Geometry check sheet. Reference: the model listing, model coordinates, mm. Face numbers are marked on the shaded views. Round coordinates to 2 decimals unless told otherwise and drop trailing zeros. Order: outer loops, then holes, each group sorted by start corner. A loop starts at its lowest first (then second) coordinate and runs counter-clockwise, first axis right, second up.
(1) Sectioned sample at C-C (z = 8). Record the boundary of the cut face in (x, y), plus the area to 3 significant figures.
(2) Sectioned sample at D-D (y = -1.95). Record the boundary of the cut face in (x, z).
(3) Material ranges on line 1 along Y through (x, z) = (8, 5.5); line 2 along X through (y, z) = (-0.45, -12); line 3 along X through (y, z) = (-0.2, 14.5), recorded low to high.
(4) Sectioned sample at A-A (y = 0). Record the boundary of the cut face in (x, z), plus the area to 3 significant figures.
(5) Sectioned sample at B-B (x = 0). Record the boundary of the cut face in (y, z).
(6) Release check for a two-part mould opening along X. For the marked faces 1 and 2 record: +X half, -X half, draft (parallel to the pull), parting line (faces both ways), or undercut.
(7) Go/stop test with flat-tipped pins: pin 1 (1 mm diameter, centred on y = 1.5, z = -7, fed in from -X); pin 2 (1.5 mm diameter, centred on x = 9.5, z = 12, fed in from -Y). Record where each tip stops, or that it passes through.
from build123d import *

# Parameters (mm, degrees)
SKETCH1_R                       = 3
BOSS_EXTRUDE1_DEPTH             = 17.5
M3_CLEARANCE_HOLE_D             = 3.2
BOSS_EXTRUDE2_REACH             = 19.5
SKETCH2_R                       = 3
BOSS_EXTRUDE2_DIRECTION_2_REACH = 19.5
M3_CLEARANCE_HOLE2_D            = 3.2


with BuildPart() as part:
    # Sketch1 → Boss-Extrude1 (new body, symmetric)
    with BuildSketch(Plane.XY):
        Circle(SKETCH1_R)
    extrude(amount=BOSS_EXTRUDE1_DEPTH, both=True)

    # M3 Clearance Hole (through all)
    with Locations(Plane.XY.offset(17.5)):
        with Locations((0, 0)):
            Hole(M3_CLEARANCE_HOLE_D / 2)

    # Boss-Extrude2: up to this face of the body (flat: up to its plane)
    boss_extrude2_end = Plane(part.part.faces().sort_by_distance((-2.915147186, 0, 17.5))[0])
    # Sketch2 → Boss-Extrude2 (add, up to the picked face)
    with BuildSketch(Plane.XY, mode=Mode.PRIVATE) as boss_extrude2_sk1:
        with Locations((8, 0)):
            Circle(SKETCH2_R)
    boss_extrude2_tool1 = split(extrude(boss_extrude2_sk1.sketch, amount=BOSS_EXTRUDE2_REACH, mode=Mode.PRIVATE), bisect_by=boss_extrude2_end, keep=Keep.BOTH, mode=Mode.PRIVATE)
    add(boss_extrude2_tool1.solids().sort_by_distance((8, 0, 0))[0])
    # Sketch2 → Boss-Extrude2 (add, up to the picked face)
    with BuildSketch(Plane.XY, mode=Mode.PRIVATE) as boss_extrude2_sk2:
        with BuildLine():
            ThreePointArc((6.02739726, -2.260273973), (5, 0), (6.02739726, 2.260273973))
            ThreePointArc((6.02739726, 2.260273973), (4, 1.5), (1.97260274, 2.260273973))
            ThreePointArc((1.97260274, 2.260273973), (2.731099432, 1.241408833), (3, 0))
            ThreePointArc((3, 0), (2.731099432, -1.241408833), (1.97260274, -2.260273973))
            ThreePointArc((1.97260274, -2.260273973), (4, -1.5), (6.02739726, -2.260273973))
        make_face()
    boss_extrude2_tool2 = split(extrude(boss_extrude2_sk2.sketch, amount=BOSS_EXTRUDE2_REACH, mode=Mode.PRIVATE), bisect_by=boss_extrude2_end, keep=Keep.BOTH, mode=Mode.PRIVATE)
    add(boss_extrude2_tool2.solids().sort_by_distance((4, 0, 0))[0])

    # Boss-Extrude2 direction 2: up to this face of the body (flat: up to its plane)
    boss_extrude2_direction_2_end = Plane(part.part.faces().sort_by_distance((-2.915147186, 0, -17.5))[0])
    # Sketch2 → Boss-Extrude2 direction 2 (add, up to the picked face)
    with BuildSketch(Plane.XY, mode=Mode.PRIVATE) as boss_extrude2_direction_2_sk1:
        with Locations((8, 0)):
            Circle(SKETCH2_R)
    boss_extrude2_direction_2_tool1 = split(extrude(boss_extrude2_direction_2_sk1.sketch, amount=-BOSS_EXTRUDE2_DIRECTION_2_REACH, mode=Mode.PRIVATE), bisect_by=boss_extrude2_direction_2_end, keep=Keep.BOTH, mode=Mode.PRIVATE)
    add(boss_extrude2_direction_2_tool1.solids().sort_by_distance((8, 0, 0))[0])
    # Sketch2 → Boss-Extrude2 direction 2 (add, up to the picked face)
    with BuildSketch(Plane.XY, mode=Mode.PRIVATE) as boss_extrude2_direction_2_sk2:
        with BuildLine():
            ThreePointArc((6.02739726, -2.260273973), (5, 0), (6.02739726, 2.260273973))
            ThreePointArc((6.02739726, 2.260273973), (4, 1.5), (1.97260274, 2.260273973))
            ThreePointArc((1.97260274, 2.260273973), (2.731099432, 1.241408833), (3, 0))
            ThreePointArc((3, 0), (2.731099432, -1.241408833), (1.97260274, -2.260273973))
            ThreePointArc((1.97260274, -2.260273973), (4, -1.5), (6.02739726, -2.260273973))
        make_face()
    boss_extrude2_direction_2_tool2 = split(extrude(boss_extrude2_direction_2_sk2.sketch, amount=-BOSS_EXTRUDE2_DIRECTION_2_REACH, mode=Mode.PRIVATE), bisect_by=boss_extrude2_direction_2_end, keep=Keep.BOTH, mode=Mode.PRIVATE)
    add(boss_extrude2_direction_2_tool2.solids().sort_by_distance((4, 0, 0))[0])

    # M3 Clearance Hole2 (through all)
    with Locations(Plane.XY.offset(17.5)):
        with Locations((8, 0)):
            Hole(M3_CLEARANCE_HOLE2_D / 2)


solid = part.part
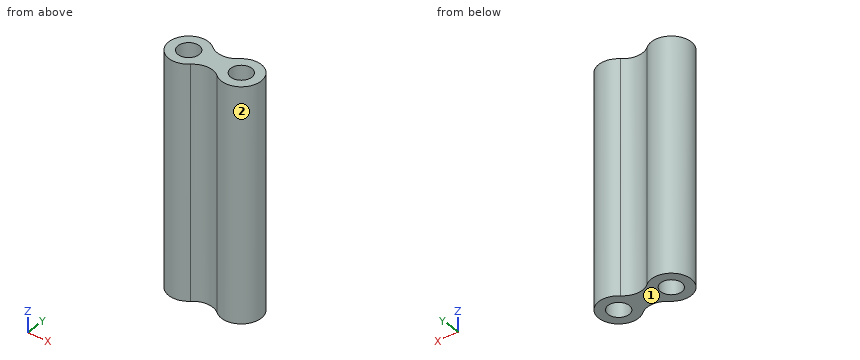
Answer below:
1. outline: (1.97, -2.26) arc R3.08 cw to (6.03, -2.26) arc R3 ccw (long way) to (6.03, 2.26) arc R3.08 cw to (1.97, 2.26) arc R3 ccw (long way) to start; hole circle Ø3.2 at (0, 0); hole circle Ø3.2 at (8, 0)
1. area: 48.1 mm2
2. outline: (-2.28, -17.5) - (2.4, -17.5) - (2.4, 17.5) - (-2.28, 17.5) - close; (5.6, -17.5) - (10.28, -17.5) - (10.28, 17.5) - (5.6, 17.5) - close
3. line 1: y = -3 to -1.6, 1.6 to 3
3. line 2: x = -2.97 to -1.54, 1.54 to 6.46, 9.54 to 10.97
3. line 3: x = -2.99 to -1.59, 1.59 to 6.41, 9.59 to 10.99
4. outline: (-3, -17.5) - (-1.6, -17.5) - (-1.6, 17.5) - (-3, 17.5) - close; (1.6, -17.5) - (6.4, -17.5) - (6.4, 17.5) - (1.6, 17.5) - close; (9.6, -17.5) - (11, -17.5) - (11, 17.5) - (9.6, 17.5) - close
4. area: 266 mm2
5. outline: (-3, -17.5) - (-1.6, -17.5) - (-1.6, 17.5) - (-3, 17.5) - close; (1.6, -17.5) - (3, -17.5) - (3, 17.5) - (1.6, 17.5) - close
6. face 1: draft
6. face 2: undercut
7. pin 1: stops at x = -2.83
7. pin 2: stops at y = -2.9
